```python
from build123d import *

# Parameters (mm, degrees)
BOSS_EXTRUDE1_DEPTH             = 5
BOSS_EXTRUDE2_REACH             = 255.229
SKETCH2_R                       = 1.25
BOSS_EXTRUDE2_DIRECTION_2_REACH = 255.229
CUT_EXTRUDE1_DEPTH              = 256.726416312
CUT_EXTRUDE1_DEPTH_BACK         = 256.726416312
SKETCH4_W                       = 20
SKETCH4_H                       = 50
SKETCH5_R                       = 11
BOSS_EXTRUDE3_DEPTH             = 12
BOSS_EXTRUDE4_DEPTH             = 7.5
FILLET1_R                       = 1


with BuildPart() as part:
    # Sketch1 → Boss-Extrude1 (new body)
    with BuildSketch(Plane(origin=(0, 0, 0), x_dir=(1, 0, 0), z_dir=(0, 1, 0))):
        Polygon((0, -40), (0, 40), (250, 10), (250, -10), align=None)
    extrude(amount=BOSS_EXTRUDE1_DEPTH)

    # Boss-Extrude2: up to this plane
    boss_extrude2_end = Plane(origin=(4.731861199, 5, 39.432176656), z_dir=(-0.11914522061843066, 0, -0.9928768384869221))
    # Sketch2 → Boss-Extrude2 (add, up to the surface)
    with BuildSketch(Plane.XY, mode=Mode.PRIVATE) as boss_extrude2_sk1:
        with BuildLine():
            Line((0, 30), (0, 5))
            Line((0, 5), (12, 5))
            Line((12, 5), (12, 30))
            ThreePointArc((12, 30), (6, 36), (0, 30))
        make_face()
        with Locations((6, 30)):
            Circle(SKETCH2_R, mode=Mode.SUBTRACT)
    boss_extrude2_tool1 = split(extrude(boss_extrude2_sk1.sketch, amount=BOSS_EXTRUDE2_REACH, mode=Mode.PRIVATE), bisect_by=boss_extrude2_end, keep=Keep.BOTH, mode=Mode.PRIVATE)
    add(boss_extrude2_tool1.solids().sort_by_distance((6, 19.745192, 0))[0])
    # Sketch2 → Boss-Extrude2 (add, up to the surface)
    with BuildSketch(Plane.XY, mode=Mode.PRIVATE) as boss_extrude2_sk2:
        with BuildLine():
            Line((238, 8), (238, 5))
            Line((238, 5), (250, 5))
            Line((250, 5), (250, 8))
            ThreePointArc((250, 8), (244, 14), (238, 8))
        make_face()
        with Locations((244, 8)):
            Circle(SKETCH2_R, mode=Mode.SUBTRACT)
    boss_extrude2_tool2 = split(extrude(boss_extrude2_sk2.sketch, amount=BOSS_EXTRUDE2_REACH, mode=Mode.PRIVATE), bisect_by=boss_extrude2_end, keep=Keep.BOTH, mode=Mode.PRIVATE)
    add(boss_extrude2_tool2.solids().sort_by_distance((244, 13.85, 0))[0])

    # Boss-Extrude2 direction 2: up to this plane
    boss_extrude2_direction_2_end = Plane(origin=(4.731861199, 5, -39.432176656), z_dir=(-0.11914522061843066, 0, 0.9928768384869221))
    # Sketch2 → Boss-Extrude2 direction 2 (add, up to the surface)
    with BuildSketch(Plane.XY, mode=Mode.PRIVATE) as boss_extrude2_direction_2_sk1:
        with BuildLine():
            Line((0, 30), (0, 5))
            Line((0, 5), (12, 5))
            Line((12, 5), (12, 30))
            ThreePointArc((12, 30), (6, 36), (0, 30))
        make_face()
        with Locations((6, 30)):
            Circle(SKETCH2_R, mode=Mode.SUBTRACT)
    boss_extrude2_direction_2_tool1 = split(extrude(boss_extrude2_direction_2_sk1.sketch, amount=-BOSS_EXTRUDE2_DIRECTION_2_REACH, mode=Mode.PRIVATE), bisect_by=boss_extrude2_direction_2_end, keep=Keep.BOTH, mode=Mode.PRIVATE)
    add(boss_extrude2_direction_2_tool1.solids().sort_by_distance((6, 19.745192, 0))[0])
    # Sketch2 → Boss-Extrude2 direction 2 (add, up to the surface)
    with BuildSketch(Plane.XY, mode=Mode.PRIVATE) as boss_extrude2_direction_2_sk2:
        with BuildLine():
            Line((238, 8), (238, 5))
            Line((238, 5), (250, 5))
            Line((250, 5), (250, 8))
            ThreePointArc((250, 8), (244, 14), (238, 8))
        make_face()
        with Locations((244, 8)):
            Circle(SKETCH2_R, mode=Mode.SUBTRACT)
    boss_extrude2_direction_2_tool2 = split(extrude(boss_extrude2_direction_2_sk2.sketch, amount=-BOSS_EXTRUDE2_DIRECTION_2_REACH, mode=Mode.PRIVATE), bisect_by=boss_extrude2_direction_2_end, keep=Keep.BOTH, mode=Mode.PRIVATE)
    add(boss_extrude2_direction_2_tool2.solids().sort_by_distance((244, 13.85, 0))[0])

    # Sketch4 → Cut-Extrude1 (cut, two sides: drawn at the far end of the back side and taken through both)
    with BuildSketch(Plane(origin=(0, 0, 0), x_dir=(1, 0, 0), z_dir=(0, 1, 0)).offset(-CUT_EXTRUDE1_DEPTH_BACK)):
        with Locations((10, 0)):
            Rectangle(SKETCH4_W, SKETCH4_H)
    extrude(amount=CUT_EXTRUDE1_DEPTH + CUT_EXTRUDE1_DEPTH_BACK, mode=Mode.SUBTRACT)

    # Sketch5 → Boss-Extrude3 (add)
    with BuildSketch(Plane.ZY.offset(-20)):
        with BuildLine():
            Line((-17.5, 30), (-17.5, 5))
            Line((-17.5, 5), (17.5, 5))
            Line((17.5, 5), (17.5, 30))
            ThreePointArc((17.5, 30), (0, 47.5), (-17.5, 30))
        make_face()
        with Locations((0, 30)):
            Circle(SKETCH5_R, mode=Mode.SUBTRACT)
    extrude(amount=-BOSS_EXTRUDE3_DEPTH)

    # Sketch6 → Boss-Extrude4 (add, symmetric)
    with BuildSketch(Plane.XY):
        with BuildLine():
            Line((200, 11), (220, 11))
            ThreePointArc((220, 11), (224, 15), (220, 19))
            Line((220, 19), (200, 19))
            ThreePointArc((200, 19), (190.100505063, 14.899494937), (186, 5))
            Line((186, 5), (194, 5))
            ThreePointArc((194, 5), (195.757359313, 9.242640687), (200, 11))
        make_face()
    extrude(amount=BOSS_EXTRUDE4_DEPTH, both=True)

    # Fillet1
    fillet1_edges = [part.edges().sort_by_distance(p)[0] for p in [
        (224, 15, -7.5),
        (210, 19, -7.5),
        (190.100505063, 14.899494937, -7.5),
        (190, 5, -7.5),
        (186, 5, 0),
        (195.757359313, 9.242640687, -7.5),
        (194, 5, 0),
        (210, 11, -7.5),
        (224, 15, 7.5),
        (210, 19, 7.5),
        (190.100505063, 14.899494937, 7.5),
        (190, 5, 7.5),
        (195.757359313, 9.242640687, 7.5),
        (210, 11, 7.5),
    ]]
    fillet(fillet1_edges, radius=FILLET1_R)


solid = part.part
```
Source: CAD feature listing. Evaluate the final solid. Frame: model axes, mm. A direction names the side the tool comes from. Round coordinates to 2 decimals unless told otherwise and drop trailing zeros. Loops run counter-clockwise (first coordinate to the right, second up) from the corner with the lowest first, then second, coordinate; pieces in that order, holes last.
(1) Section query B-B (y = 25.5). Output: boundary loops of the cut face in (x, z), and give its area (3 significant figures).
From the geometry:
outline: (0, -40) - (12, -38.56) - (12, -25) - (0, -25) - close; (0, 25) - (12, 25) - (12, 38.56) - (0, 40) - close; (20, -17.5) - (32, -17.5) - (32, -10.04) - (20, -10.04) - close; (20, 10.04) - (32, 10.04) - (32, 17.5) - (20, 17.5) - close
area: 522 mm2
(2) Contact query for flat-ended pins moving along their axis: pin 1 Ø10 at (x, y) = (8.5, 12.5) entering from -Z; pin 2 Ø7 at (y, z) = (13.5, -28.5) entering from +X; pin 3 Ø0.9 at (y, z) = (6.5, 5) entering from -X. Output: stop coordinate, or through.
From the geometry:
pin 1: stops at z = -39.58
pin 2: stops at x = 12
pin 3: stops at x = 20
(3) Section query D-D (x = 231.5). Output: boundary loops of the cut face in (y, z).
From the geometry:
outline: (0, -12.22) - (5, -12.22) - (5, 12.22) - (0, 12.22) - close
(4) Material intervals for probe 1 along X at (y, z) = (8, 9); probe 2 along X at (y, z) = (8, -1); probe 3 along X at (y, z) = (30, 33.5), sorted ascending.
From the geometry:
probe 1: x = 20 to 32, 238 to 242.75, 245.25 to 250
probe 2: x = 20 to 32, 186.33 to 194.8, 238 to 242.75, 245.25 to 250
probe 3: x = 0 to 4.75, 7.25 to 12
(5) Access query for faces 1 (the flat face through (210, 11, 0)), 2 (the flat face through (5, 18, -25)), 3 (the cylindrical face through (190.54, 15.32, 0.09)), 4 (the flat face through (26, 18, -17.5)). Directions: +Z, -Z, +X, -X, +Y, -Y. A direction counts if a zero-diameter tool reaches every point of the face in a straight line with its end or side. Return the directions, or none.
From the geometry:
face 1: +Z, -Z
face 2: -X, +Y, -Y
face 3: +Z, -Z, +Y
face 4: -Z, +X, -X, +Y
(6) Section query C-C (z = -33). Output: boundary loops of the cut face in (x, y), and give its area (3 significant figures).
From the geometry:
outline: (0, 0) - (58.33, 0) - (58.33, 5) - (12, 5) - (12, 30) arc R6 ccw to (0, 30) - close; hole circle Ø2.5 at (6, 30)
area: 643 mm2
(7) Section query A-A (z = 0). Output: boundary loops of the cut face in (x, y), and give its area (3 significant figures).
From the geometry:
outline: (20, 0) - (250, 0) - (250, 8) arc R6 ccw to (238, 8) - (238, 5) - (195.1, 5) arc R1 cw to (194.12, 6.2) arc R6 cw to (200, 11) - (220, 11) arc R4 ccw to (220, 19) - (200, 19) arc R14 ccw to (186.03, 5.93) arc R1 cw to (185.03, 5) - (32, 5) - (32, 19) - (20, 19) - close; (20, 41) - (32, 41) - (32, 47.5) - (20, 47.5) - close; hole circle Ø2.5 at (244, 8)
area: 1,790 mm2
(8) Pull-direction query (X, two-part tool) for faces 5 (the cylindrical face through (224, 15, 0)), 6 (the flat face through (12, 17, 32)), 7 (the cylindrical face through (25.92, 19.26, -2.38)), 8 (the flat face through (32, 17, 0)); classes: +X half, -X half, draft (parallel to the pull), parting line (faces both ways), or undercut.
From the geometry:
face 5: undercut
face 6: +X half
face 7: draft
face 8: undercut
